```python
from build123d import *

# Parameters (mm, degrees)
ESQUISSE1_W             = 200
ESQUISSE1_H             = 155
BOSS_EXTRU_1_DEPTH      = 5
ENL_V_MAT_EXTRU_1_DEPTH = 127.614572621
ESQUISSE4_W             = 200
ESQUISSE4_H             = 5
BOSS_EXTRU_2_DEPTH      = 42
CONG_1_R                = 60
ESQUISSE5_R             = 1.5
ENL_V_MAT_EXTRU_2_DEPTH = 17


with BuildPart() as part:
    # Esquisse1 → Boss.-Extru.1 (new body)
    with BuildSketch(Plane.XY):
        Rectangle(ESQUISSE1_W, ESQUISSE1_H)
    extrude(amount=BOSS_EXTRU_1_DEPTH)

    # Esquisse2 → Enlèv. mat.-Extru.1 (cut, through all)
    with BuildSketch(Plane.XY.offset(5)):
        Polygon((-96, 37.883974596), (-96, 39.616025404), (-97.5, 40.482050808), (-99, 39.616025404), (-99, 37.883974596), (-97.5, 37.017949192), align=None)
        Polygon((-97.5, -37.017949192), (-96, -37.883974596), (-96, -39.616025404), (-97.5, -40.482050808), (-99, -39.616025404), (-99, -37.883974596), align=None)
        Polygon((99, -37.883974596), (97.5, -37.017949192), (96, -37.883974596), (96, -39.616025404), (97.5, -40.482050808), (99, -39.616025404), align=None)
        Polygon((97.5, 37.017949192), (96, 37.883974596), (96, 39.616025404), (97.5, 40.482050808), (99, 39.616025404), (99, 37.883974596), align=None)
        Polygon((-51, -75.866025404), (-51, -74.133974596), (-52.5, -73.267949192), (-54, -74.133974596), (-54, -75.866025404), (-52.5, -76.732050808), align=None)
        Polygon((52.5, -76.732050808), (51, -75.866025404), (51, -74.133974596), (52.5, -73.267949192), (54, -74.133974596), (54, -75.866025404), align=None)
    extrude(amount=-ENL_V_MAT_EXTRU_1_DEPTH, mode=Mode.SUBTRACT)

    # Esquisse4 → Boss.-Extru.2 (add)
    with BuildSketch(Plane(origin=(0, 77.5, 0), x_dir=(1, 0, 0), z_dir=(0, 1, 0))):
        with Locations((0, -2.5)):
            Rectangle(ESQUISSE4_W, ESQUISSE4_H)
    extrude(amount=BOSS_EXTRU_2_DEPTH)

    # Congé1
    cong_1_edges = [part.edges().sort_by_distance(p)[0] for p in [
        (100, 119.5, 2.5),
        (-100, 119.5, 2.5),
    ]]
    fillet(cong_1_edges, radius=CONG_1_R)

    # Esquisse5 → Enlèv. mat.-Extru.2 (cut)
    with BuildSketch(Plane(origin=(0, 0, 0), x_dir=(-1, 0, 0), z_dir=(0, 0, -1))):
        with Locations((-9.8, 66.447157523)):
            Circle(ESQUISSE5_R)
        with Locations((0.2, 66.447157523)):
            Circle(ESQUISSE5_R)
        with Locations((-9.8, 114.447157523)):
            Circle(ESQUISSE5_R)
        with Locations((0.2, 114.447157523)):
            Circle(ESQUISSE5_R)
    extrude(amount=-ENL_V_MAT_EXTRU_2_DEPTH, mode=Mode.SUBTRACT)


solid = part.part
```
The model under review builds one solid part; all positions refer to its coordinate system, in mm. Round coordinates to 2 decimals unless told otherwise and drop trailing zeros. Loops run counter-clockwise (first coordinate to the right, second up) from the corner with the lowest first, then second, coordinate; pieces in that order, holes last. Notation, with made-up numbers: M -31.5,64.25 L -14.5,64.25 A31 ccw -14.5,101.25 Z; hole C -10.75,-24.5 d6. An arc over 180 degrees is marked long. Write item = value, one per line.
Item 1: Take a section at B-B on x = 65.5. Write out the cut boundary in (y, z).
Return value:
outline = M -77.5,0 L 113.81,0 L 113.81,5 L -77.5,5 Z
Item 2: Take a section at A-A on z = 1.3. State how many separate pieces and enclosed holes the cut face has, then the cut area to 3 significant figures.
Return value:
separate_pieces = 1
enclosed_holes = 10
area = 37,800 mm2
Item 3: Insertion check: P1, Ø2.5, axis at x = -0.2, y = 114.45, coming from the +Z side. The pin has a flat end and moves straight along its axis. Give the tip position at first contact, or say it passes through.
Return value:
P1 = through
Item 4: For line 1 (Y direction, x = -0.2, z = 2.7); line 2 (X direction, y = 67.5, z = 3.05); line 3 (X direction, y = 66, z = 1.7), list the stretches that pass through material, from the lowest coordinate up. Write a range as [from, to].
Return value:
line_1 = [-77.5, 64.95], [67.95, 112.95], [115.95, 119.5]
line_2 = [-99.46, -1.27], [0.87, 8.73], [10.87, 99.46]
line_3 = [-99.65, -1.63], [1.23, 8.37], [11.23, 99.65]
Item 5: Take a section at C-C on y = 83. Write out the cut boundary in (x, z).
Return value:
outline = M -95.21,0 L 95.21,0 L 95.21,5 L -95.21,5 Z
